The listing builds one solid part. Answer for the finished solid, in the listing's coordinates (mm). Face numbers are marked on the shaded views. A direction names the side the tool comes from. Coordinates: 2 decimals unless noted, no trailing zeros. Loops run counter-clockwise (first coordinate to the right, second up) from the corner with the lowest first, then second, coordinate; pieces in that order, holes last. Notation, with made-up numbers: (-27, 45) -> (21, 45) arc R18 ccw to (21, 72) -> close; hole circle Ø1 at (21.5, 12.5). An arc over 180 degrees is marked (long way). Answer in a Markdown table with one row per item.
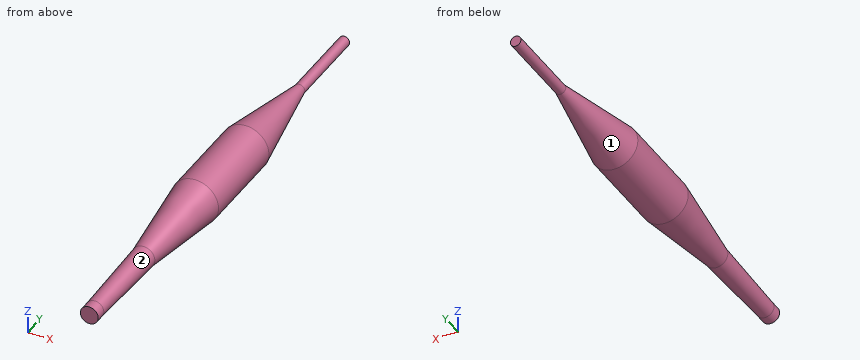
```python
from build123d import *

# Parameters (mm, degrees)
F0_W   = 25
F0_H   = 21
F0_W_2 = 224.9109574539
F0_H_2 = 55
F0_W_3 = 200
F0_H_3 = 12.5


# Not quite as in the source:
# - the program builds the solid bodies; features that only make, move or delete a surface that nothing else refers to are left out


with BuildPart() as f1:
    # F0 (on Right) → F1 (revolve)
    with BuildSketch(Plane.YZ):
        with Locations((12.5, 223.4762815751)):
            Rectangle(F0_W, F0_H)
        Polygon((25, 233.9762815751), (25, 212.9762815751), (242, 212.9762815751), (242, 239.6586265556), align=None)
        Polygon((242, 239.6586265556), (242, 212.9762815751), (344.0616714118, 212.9762815751), (344.0616714118, 252.1902240649), align=None)
        Polygon((344.0616714118, 252.1902240649), (344.0616714118, 212.9762815751), (472.6287925066, 212.9762815751), (472.6287925066, 267.9762815751), align=None)
        with Locations((585.0842712335, 240.4762815751)):
            Rectangle(F0_W_2, F0_H_2)
        Polygon((697.5397499605, 267.9762815751), (697.5397499605, 212.9762815751), (853.5, 212.9762815751), (853.5, 240.4762815751), align=None)
        Polygon((853.5, 240.4762815751), (853.5, 212.9762815751), (938.5692272943, 212.9762815751), (938.5692272943, 225.4762815751), align=None)
        with Locations((1038.5692272943, 219.2262815751)):
            Rectangle(F0_W_3, F0_H_3)
    revolve(axis=Axis((0, -32.5, 212.9762815751), (0, -1, 0)))


solid = f1.part
```
Item 1: A tool of negligible diameter and unlimited length cuts with its end or side. For the marked faces 1 and 2, from which of +Z, -Z, +X, -X, +Y, -Y can it reach the whole face along a straight path? Write none if from no direction.
Findings below:
| item | result |
|---|---|
| face 1 | +Y |
| face 2 | -Y |
Item 2: Find the intervals of material crossed by probe 1 along Z at (x, y) = (2, 637.5); probe 2 along Z at (x, y) = (-48, 514.5); probe 3 along X at (y, z) = (659.5, 194), in increasing order.
Findings below:
| item | result |
|---|---|
| probe 1 | z = 158.01 to 267.94 |
| probe 2 | z = 186.12 to 239.83 |
| probe 3 | x = -51.62 to 51.62 |
Item 3: Flat-ended cylindrical pins translate along their axes: pin 1 Ø2 at (y, z) = (949.5, 220) entering from -X; pin 2 Ø6 at (x, y) = (-17.5, 916.5) entering from -Z; pin 3 Ø1 at (y, z) = (835, 244.5) entering from -X. Find the tip coordinate at first contact, or state that the pin passes through.
Findings below:
| item | result |
|---|---|
| pin 1 | stops at x = -10.95 |
| pin 2 | stops at z = 205.22 |
| pin 3 | passes through |
Item 4: A cutting plane is placed at A-A, the plane x = 0. Determine the outline of the cut face in (y, z).
Findings below:
| item | result |
|---|---|
| outline | (0, 191.98) -> (25, 191.98) -> (242, 186.29) -> (472.63, 157.98) -> (697.54, 157.98) -> (938.57, 200.48) -> (1138.57, 200.48) -> (1138.57, 225.48) -> (938.57, 225.48) -> (697.54, 267.98) -> (472.63, 267.98) -> (242, 239.66) -> (25, 233.98) -> (0, 233.98) -> close |
Item 5: A cutting plane is placed at B-B, the plane y = 650. Determine the outline of the cut face in (x, z).
Findings below:
| item | result |
|---|---|
| outline | circle Ø110 at (0, 212.98) |
Item 6: A cutting plane is placed at C-C, the plane y = 990. Determine the outline of the cut face in (x, z).
Findings below:
| item | result |
|---|---|
| outline | circle Ø25 at (0, 212.98) |
